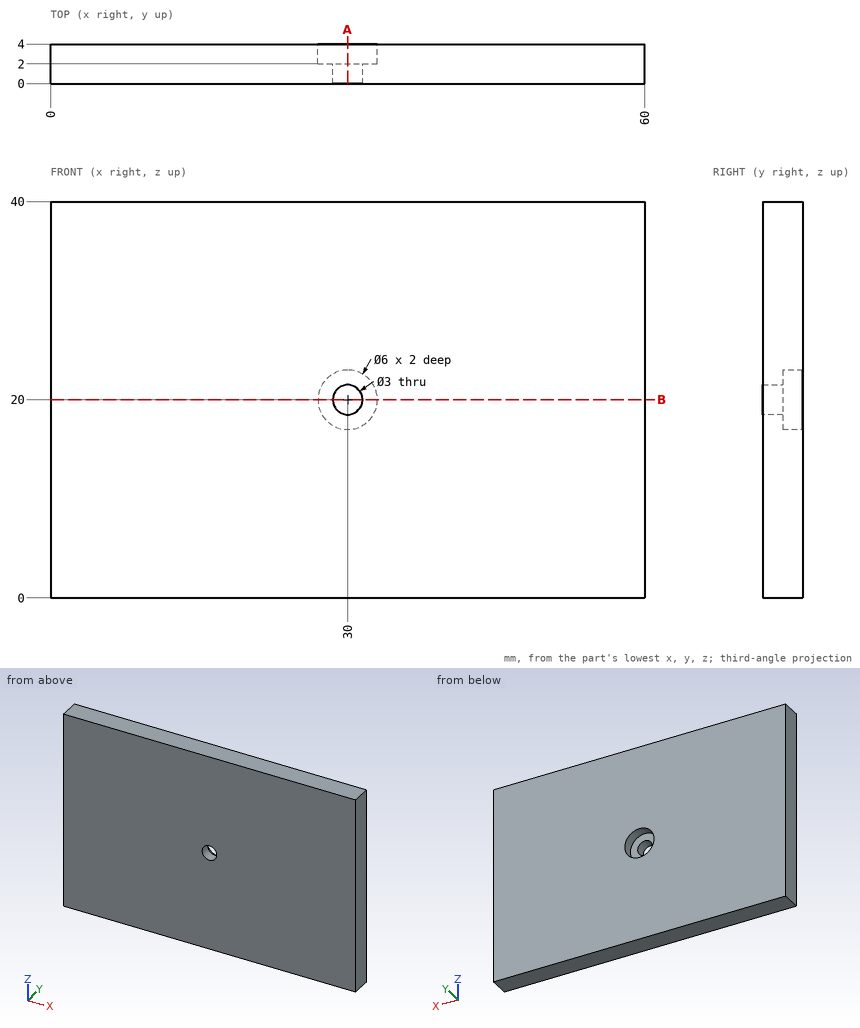
Check sheet for the drawn part. Datum: minimum x, y, z corner. Units: mm. Coordinates: 2 decimals unless noted, no trailing zeros. Order: outer loops, then holes, each group sorted by start corner. A loop starts at its lowest first (then second) coordinate and runs counter-clockwise, first axis right, second up. Notation, with made-up numbers: (54.5, 4.5) - (105.5, 4.5) arc R31 ccw to (105.5, 32.5) - close; hole circle Ø11 at (50, -39). An arc over 180 degrees is marked (long way). Return JSON: item names as keys, results as strings.
(1) Section check B-B, the plane z = 20. Record the cut outline in (x, y), and give its area (3 significant figures).
Filled sheet:
{"outline": "(0, 0) - (28.5, 0) - (28.5, 2) - (27, 2) - (27, 4) - (0, 4) - close; (31.5, 0) - (60, 0) - (60, 4) - (33, 4) - (33, 2) - (31.5, 2) - close", "area": "222 mm^2"}
(2) Go/stop test with flat-tipped pins: pin 1 (1.8 mm diameter, centred on x = 30, z = 20, fed in from +Y); pin 2 (3.5 mm diameter, centred on x = 30, z = 20, fed in from +Y). Record where each tip stops, or that it passes through.
Filled sheet:
{"pin 1": "passes through", "pin 2": "stops at y = 2"}
(3) Section check A-A, the plane x = 30. Record the cut outline in (y, z), and give its area (3 significant figures).
Filled sheet:
{"outline": "(0, 0) - (4, 0) - (4, 17) - (2, 17) - (2, 18.5) - (0, 18.5) - close; (0, 21.5) - (2, 21.5) - (2, 23) - (4, 23) - (4, 40) - (0, 40) - close", "area": "142 mm^2"}
(4) Thickness scan on line 1 along X through (y, z) = (0.5, 20); line 2 along X through (y, z) = (3.35, 20); line 3 along Z through (x, y) = (30, 2.95). Record the ranges inside material, lowest first.
Filled sheet:
{"line 1": "x = 0 to 28.5, 31.5 to 60", "line 2": "x = 0 to 27, 33 to 60", "line 3": "z = 0 to 17, 23 to 40"}
